The listing builds one solid part. Answer for the finished solid, in the listing's coordinates (mm). Face numbers are marked on the shaded views. A direction names the side the tool comes from. Give positions to 0.01 mm unless a question says otherwise; leave off trailing zeros. Write each loop counter-clockwise with the first axis right and the second up, starting at its lowest first coordinate (ties: lowest second). Pieces come first, ordered by that corner, then holes. Notation, with made-up numbers: (50, -3.5) -> (93, -3.5) arc R33 ccw to (93, 27.5) -> close; hole circle Ø10 at (23.5, 41.25). An arc over 180 degrees is marked (long way). Put each result on its own line as item: value. Start each with the question number.
1) A cutting plane is placed at D-D (z = 0). Give the number of separate pieces and of enclosed holes in the cut face, then the cut area to 3 significant figures.
2) A cutting plane is placed at A-A (x = -18.75). Write down the section's boundary in (y, z) (3 decimals), then the cut area to 3 significant figures.
3) Find the intervals of material crossed by line 1 along Z through (x, y) = (0, 6.55) (3 decimals); line 2 along X through (y, z) = (6.4, 18.75); line 3 along Z through (x, y) = (-20.25, 12.5) (3 decimals), in increasing order. Write a range as from..to.
4) A cutting plane is placed at C-C (z = 18). Write down the section's boundary in (x, y), then the cut area to 3 significant figures.
5) Flat-ended cylindrical pins translate along their axes: pin 1 Ø5 at (x, z) = (-31, 8) entering from -Y; pin 2 Ø3 at (x, y) = (-3.5, 10.5) entering from +Z; pin 3 Ø2 at (y, z) = (10, 21.5) entering from +X; pin 4 Ø4.5 at (y, z) = (12.5, 0) entering from +X (3 decimals). Find the tip coordinate at first contact, or state that the pin passes through.
6) For a pull along X with two mould halves and no side action, classify the marked faces 5, 6, 7 and 8 as released by +X, released by -X, zero draft, split by the parting line, or undercut.
7) A cutting plane is placed at B-B (y = 8.75). Write down the section's boundary in (x, z) (3 decimals).
8) For the marked faces 1, 2, 3 and 4, determine the directions among +Z, -Z, +X, -X, +Y, -Y from which every point of the face is accessible in a straight line to the end or side of a thin tool.
from build123d import *

# Parameters (mm, degrees)
SKETCH1_W                      = 60
SKETCH1_H                      = 57
BOSS_EXTRUDE1_DEPTH            = 7.5
SKETCH3_R                      = 8.75
SKETCH3_R_2                    = 5.175
BOSS_EXTRUDE2_DEPTH            = 10
CUT_EXTRUDE1_START             = -4.5
SKETCH4_R                      = 5.175
CUT_EXTRUDE1_DEPTH             = 4.5
CBORE_FOR_M3_SHCS2_D           = 4.25
CBORE_FOR_M3_SHCS2_DEPTH       = 10
CBORE_FOR_M3_SHCS2_CBORE_D     = 5.25
CBORE_FOR_M3_SHCS2_CBORE_DEPTH = 0.5
SKETCH_PATTERN1_START          = 3
SKETCH_PATTERN1_OUTLINE_R      = 5.175
SKETCH_PATTERN1_DEPTH          = 4.5
SKETCH_PATTERN1_START_2        = 15.125
SKETCH_PATTERN1_2_OUTLINE_R    = 5.175
SKETCH_PATTERN1_2_DEPTH        = 2.375
SKETCH_PATTERN1_START_3        = 7.5
SKETCH_PATTERN1_3_OUTLINE_R    = 5.175
SKETCH_PATTERN1_3_DEPTH        = 2.3749999
SKETCH_PATTERN1_START_4        = 9.8749999
SKETCH_PATTERN1_4_OUTLINE_R    = 5.175
SKETCH_PATTERN1_4_DEPTH        = 5.2500001
SKETCH_PATTERN1_START_5        = -24
SKETCH_PATTERN1_5_OUTLINE_R    = 2.125
SKETCH_PATTERN1_5_DEPTH        = 8.05
SKETCH_PATTERN1_START_6        = 4.718580183
SKETCH_PATTERN1_6_OUTLINE_R    = 2.125
SKETCH_PATTERN1_6_DEPTH        = 7.456419817
SKETCH_PATTERN1_START_7        = -16.45
SKETCH_PATTERN1_7_OUTLINE_R    = 2.625
SKETCH_PATTERN1_7_OUTLINE_R_2  = 2.125
SKETCH_PATTERN1_7_DEPTH        = 0.5
SKETCH_PATTERN1_START_8        = 11.675
SKETCH_PATTERN1_8_OUTLINE_R    = 2.625
SKETCH_PATTERN1_8_OUTLINE_R_2  = 2.125
SKETCH_PATTERN1_8_DEPTH        = 0.5
CBORE_FOR_M3_SHCS1_D           = 3.4
CBORE_FOR_M3_SHCS1_CBORE_D     = 6.5
CBORE_FOR_M3_SHCS1_CBORE_DEPTH = 3
FILLET2_R                      = 3


with BuildPart() as part:
    # Sketch1 → Boss-Extrude1 (new body)
    with BuildSketch(Plane(origin=(0, 0, 0), x_dir=(1, 0, 0), z_dir=(0, 1, 0))):
        with Locations((-12.0625, 0)):
            Rectangle(SKETCH1_W, SKETCH1_H)
    extrude(amount=BOSS_EXTRUDE1_DEPTH)

    # Sketch3 → Boss-Extrude2 (add)
    # profile 1 of 2: a face of its own
    with BuildSketch(Plane(origin=(0, 7.5, 0), x_dir=(1, 0, 0), z_dir=(0, 1, 0))):
        with Locations((-28.125, 18.75)):
            Circle(SKETCH3_R)
        with Locations(Location((-28.125, 18.75, 0), (0, 0, 270))):
            Circle(SKETCH3_R_2, mode=Mode.SUBTRACT)
    # profile 2 of 2: a face of its own
    with BuildSketch(Plane(origin=(0, 7.5, 0), x_dir=(1, 0, 0), z_dir=(0, 1, 0))):
        with BuildLine():
            Line((-15.95, 27.5), (-28.125, 27.5))
            ThreePointArc((-28.125, 27.5), (-21.937815665, 24.937184335), (-19.375, 18.75))
            ThreePointArc((-19.375, 18.75), (-21.937815665, 12.562815665), (-28.125, 10))
            Line((-28.125, 10), (-15.95, 10))
            Line((-15.95, 10), (-15.95, 27.5))
        make_face()
    extrude(amount=BOSS_EXTRUDE2_DEPTH)

    # Sketch4 → Cut-Extrude1 (cut)
    with BuildSketch(Plane(origin=(0, 7.5, 0), x_dir=(1, 0, 0), z_dir=(0, 1, 0)).offset(CUT_EXTRUDE1_START)):
        with Locations(Location((-28.125, 18.75, 0), (0, 0, 270))):
            Circle(SKETCH4_R)
    extrude(amount=CUT_EXTRUDE1_DEPTH, mode=Mode.SUBTRACT)

    # CBORE for M3 SHCS2
    with Locations(Plane(origin=(-15.95, 0, 0), x_dir=(0, 0, -1), z_dir=(1, 0, 0))):
        with Locations((18.75, 12.5)):
            CounterBoreHole(CBORE_FOR_M3_SHCS2_D / 2, CBORE_FOR_M3_SHCS2_CBORE_D / 2, CBORE_FOR_M3_SHCS2_CBORE_DEPTH, depth=CBORE_FOR_M3_SHCS2_DEPTH)

    # Sketch-Pattern1: read off the stored shape, not the designer's step
    # Sketch-Pattern1 outline → Sketch-Pattern1 (cut)
    with BuildSketch(Plane(origin=(0, 0, 0), x_dir=(1, 0, 0), z_dir=(0, 1, 0)).offset(SKETCH_PATTERN1_START)):
        Circle(SKETCH_PATTERN1_OUTLINE_R)
        with Locations((-28.125, -18.75)):
            Circle(SKETCH_PATTERN1_OUTLINE_R)
    extrude(amount=SKETCH_PATTERN1_DEPTH, mode=Mode.SUBTRACT)

    # Sketch-Pattern1 3 outline → Sketch-Pattern1 3 (add)
    # profile 1 of 2: a face of its own
    with BuildSketch(Plane(origin=(0, 0, 0), x_dir=(1, 0, 0), z_dir=(0, 1, 0)).offset(SKETCH_PATTERN1_START_3)):
        with BuildLine():
            Line((-28.125, -27.5), (-15.95, -27.5))
            Line((-15.95, -27.5), (-15.95, -10))
            Line((-15.95, -10), (-28.125, -10))
            ThreePointArc((-28.125, -10), (-36.875, -18.75), (-28.125, -27.5))
        make_face()
        with Locations((-28.125, -18.75)):
            Circle(SKETCH_PATTERN1_3_OUTLINE_R, mode=Mode.SUBTRACT)
    # profile 2 of 2: a face of its own
    with BuildSketch(Plane(origin=(0, 0, 0), x_dir=(1, 0, 0), z_dir=(0, 1, 0)).offset(SKETCH_PATTERN1_START_3)):
        with BuildLine():
            ThreePointArc((0, 8.75), (-8.75, 0), (0, -8.75))
            Line((0, -8.75), (12.175, -8.75))
            Line((12.175, -8.75), (12.175, 8.75))
            Line((12.175, 8.75), (0, 8.75))
        make_face()
        Circle(SKETCH_PATTERN1_3_OUTLINE_R, mode=Mode.SUBTRACT)
    extrude(amount=SKETCH_PATTERN1_3_DEPTH)



with BuildPart() as body_2:
    # Sketch-Pattern1 2 outline → Sketch-Pattern1 2 (new body)
    # profile 1 of 2: a face of its own
    with BuildSketch(Plane(origin=(0, 0, 0), x_dir=(1, 0, 0), z_dir=(0, 1, 0)).offset(SKETCH_PATTERN1_START_2)):
        with BuildLine():
            Line((-28.125, -27.5), (-15.95, -27.5))
            Line((-15.95, -27.5), (-15.95, -10))
            Line((-15.95, -10), (-28.125, -10))
            ThreePointArc((-28.125, -10), (-36.875, -18.75), (-28.125, -27.5))
        make_face()
        with Locations((-28.125, -18.75)):
            Circle(SKETCH_PATTERN1_2_OUTLINE_R, mode=Mode.SUBTRACT)
    # profile 2 of 2: a face of its own
    with BuildSketch(Plane(origin=(0, 0, 0), x_dir=(1, 0, 0), z_dir=(0, 1, 0)).offset(SKETCH_PATTERN1_START_2)):
        with BuildLine():
            ThreePointArc((0, 8.75), (-8.75, 0), (0, -8.75))
            Line((0, -8.75), (12.175, -8.75))
            Line((12.175, -8.75), (12.175, 8.75))
            Line((12.175, 8.75), (0, 8.75))
        make_face()
        Circle(SKETCH_PATTERN1_2_OUTLINE_R, mode=Mode.SUBTRACT)
    extrude(amount=SKETCH_PATTERN1_2_DEPTH)


with BuildPart() as part_1:
    add(part.part)

    add(body_2.part)  # Sketch-Pattern1 4 merges body 2
    # Sketch-Pattern1 4 outline → Sketch-Pattern1 4 (add)
    # profile 1 of 2: a face of its own
    with BuildSketch(Plane(origin=(0, 0, 0), x_dir=(1, 0, 0), z_dir=(0, 1, 0)).offset(SKETCH_PATTERN1_START_4)):
        with BuildLine():
            Line((-28.125, -27.5), (-15.95, -27.5))
            Line((-15.95, -27.5), (-15.95, -10))
            Line((-15.95, -10), (-28.125, -10))
            ThreePointArc((-28.125, -10), (-36.875, -18.75), (-28.125, -27.5))
        make_face()
        with Locations((-28.125, -18.75)):
            Circle(SKETCH_PATTERN1_4_OUTLINE_R, mode=Mode.SUBTRACT)
    # profile 2 of 2: a face of its own
    with BuildSketch(Plane(origin=(0, 0, 0), x_dir=(1, 0, 0), z_dir=(0, 1, 0)).offset(SKETCH_PATTERN1_START_4)):
        with BuildLine():
            ThreePointArc((0, 8.75), (-8.75, 0), (0, -8.75))
            Line((0, -8.75), (12.175, -8.75))
            Line((12.175, -8.75), (12.175, 8.75))
            Line((12.175, 8.75), (0, 8.75))
        make_face()
        Circle(SKETCH_PATTERN1_4_OUTLINE_R, mode=Mode.SUBTRACT)
    extrude(amount=SKETCH_PATTERN1_4_DEPTH)

    # Sketch-Pattern1 5 outline → Sketch-Pattern1 5 (cut)
    with BuildSketch(Plane.YZ.offset(SKETCH_PATTERN1_START_5)):
        with Locations((12.5, 18.75)):
            Circle(SKETCH_PATTERN1_5_OUTLINE_R)
    extrude(amount=SKETCH_PATTERN1_5_DEPTH, mode=Mode.SUBTRACT)

    # Sketch-Pattern1 6 outline → Sketch-Pattern1 6 (cut)
    with BuildSketch(Plane.YZ.offset(SKETCH_PATTERN1_START_6)):
        with Locations((12.5, 0)):
            Circle(SKETCH_PATTERN1_6_OUTLINE_R)
    extrude(amount=SKETCH_PATTERN1_6_DEPTH, mode=Mode.SUBTRACT)

    # Sketch-Pattern1 7 outline → Sketch-Pattern1 7 (cut)
    with BuildSketch(Plane.YZ.offset(SKETCH_PATTERN1_START_7)):
        with Locations((12.5, 18.75)):
            Circle(SKETCH_PATTERN1_7_OUTLINE_R)
        with Locations((12.5, 18.75)):
            Circle(SKETCH_PATTERN1_7_OUTLINE_R_2, mode=Mode.SUBTRACT)
    extrude(amount=SKETCH_PATTERN1_7_DEPTH, mode=Mode.SUBTRACT)

    # Sketch-Pattern1 8 outline → Sketch-Pattern1 8 (cut)
    with BuildSketch(Plane.YZ.offset(SKETCH_PATTERN1_START_8)):
        with Locations((12.5, 0)):
            Circle(SKETCH_PATTERN1_8_OUTLINE_R)
        with Locations((12.5, 0)):
            Circle(SKETCH_PATTERN1_8_OUTLINE_R_2, mode=Mode.SUBTRACT)
    extrude(amount=SKETCH_PATTERN1_8_DEPTH, mode=Mode.SUBTRACT)

    # CBORE for M3 SHCS1 (through all)
    with Locations(Plane(origin=(0, 7.5, 0), x_dir=(1, 0, 0), z_dir=(0, 1, 0))):
        with Locations((-37.5, 0), (0, 18.75), (-18.75, 0), (0, -18.75)):
            CounterBoreHole(CBORE_FOR_M3_SHCS1_D / 2, CBORE_FOR_M3_SHCS1_CBORE_D / 2, CBORE_FOR_M3_SHCS1_CBORE_DEPTH)

    # Fillet2
    fillet2_edges = [part_1.edges().sort_by_distance(p)[0] for p in [
        (-42.0625, 3.75, -28.5),
        (17.9375, 3.75, -28.5),
        (17.9375, 3.75, 28.5),
        (-42.0625, 3.75, 28.5),
    ]]
    fillet(fillet2_edges, radius=FILLET2_R)


solid = part_1.part
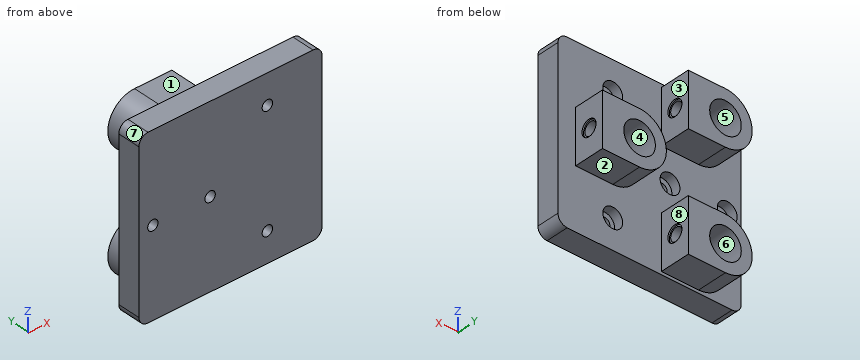
Reply:
1. separate pieces: 4
1. enclosed holes: 0
1. area: 409 mm2
2. outline: (0, -28.5) -> (7.5, -28.5) -> (7.5, -27.5) -> (17.5, -27.5) -> (17.5, -10) -> (7.5, -10) -> (7.5, -3.25) -> (4.5, -3.25) -> (4.5, -1.7) -> (0, -1.7) -> close; (0, 1.7) -> (4.5, 1.7) -> (4.5, 3.25) -> (7.5, 3.25) -> (7.5, 10) -> (17.5, 10) -> (17.5, 27.5) -> (7.5, 27.5) -> (7.5, 28.5) -> (0, 28.5) -> close; hole circle Ø4.25 at (12.5, -18.75); hole circle Ø4.25 at (12.5, 18.75)
2. area: 714 mm2
3. line 1: z = -28.5..-22, -15.5..-5.175, 5.175..15.5, 22..28.5
3. line 2: x = -42.06..-33.3, -22.95..-3.25, 3.25..17.94
3. line 3: z = -27.5..-20.875, -16.625..-10, 10..16.625, 20.875..27.5
4. outline: (-42.06, 0) -> (-1.53, 0) -> (-1.53, 4.5) -> (-3.16, 4.5) -> (-3.16, 7.5) -> (-15.95, 7.5) -> (-15.95, 9.98) -> (-16.45, 9.98) -> (-16.45, 10.51) -> (-23, 10.51) -> (-23, 3) -> (-33.25, 3) -> (-33.25, 17.5) -> (-36.84, 17.5) -> (-36.84, 7.5) -> (-42.06, 7.5) -> close; (-23, 14.49) -> (-16.45, 14.49) -> (-16.45, 15.02) -> (-15.95, 15.02) -> (-15.95, 17.5) -> (-23, 17.5) -> close; (1.53, 0) -> (17.94, 0) -> (17.94, 7.5) -> (3.16, 7.5) -> (3.16, 4.5) -> (1.53, 4.5) -> close
4. area: 449 mm2
5. pin 1: stops at y = 0
5. pin 2: stops at z = 8.52
5. pin 3: stops at x = -15.95
5. pin 4: stops at x = 11.675
6. face 5: undercut
6. face 6: undercut
6. face 7: released by -X
6. face 8: released by +X
7. outline: (-28.125, -27.5) -> (-15.95, -27.5) -> (-15.95, -10) -> (-28.125, -10) arc R8.75 ccw to start; (-28.125, 10) -> (-15.95, 10) -> (-15.95, 27.5) -> (-28.125, 27.5) arc R8.75 ccw to start; (0, -8.75) -> (12.175, -8.75) -> (12.175, 8.75) -> (0, 8.75) arc R8.75 ccw to start; hole circle Ø10.35 at (-28.125, -18.75); hole circle Ø10.35 at (-28.125, 18.75); hole circle Ø10.35 at (0, 0)
8. face 1: +Z, +X, -X, +Y
8. face 2: -Z, +X, -X, +Y
8. face 3: +Z, -Z, +X, +Y
8. face 4: +Y
